from build123d import *

# Parameters (mm, degrees)
BOSS_EXTRUDE1_DEPTH = 13.85


with BuildPart() as part:
    # Sketch1 → Boss-Extrude1 (new, symmetric)
    with BuildSketch(Plane(origin=(0, 0, 0), x_dir=(0, 0, -1), z_dir=(1, 0, 0))):
        with BuildLine():
            ThreePointArc((74.3, 0), (67.119640803, -31.866029224), (46.966384428, -57.572986146))
            Line((46.966384428, -57.572986146), (47.463876439, -58.070478157))
            ThreePointArc((47.463876439, -58.070478157), (67.76721454, -32.13416614), (75, 0))
            ThreePointArc((75, 0), (50.311529494, 55.621488653), (-7.5, 74.624057783))
            Line((-7.5, 74.624057783), (-7.5, 73.920497834))
            ThreePointArc((-7.5, 73.920497834), (49.815860928, 55.125946704), (74.3, 0))
        make_face()
    extrude(amount=BOSS_EXTRUDE1_DEPTH, both=True)


solid = part.part
For this review, take the finished solid that the model builds, in its own axes (mm). Round coordinates to 2 decimals unless told otherwise and drop trailing zeros. Order: outer loops, then holes, each group sorted by start corner. A loop starts at its lowest first (then second) coordinate and runs counter-clockwise, first axis right, second up. Notation, with made-up numbers: (80, 42.5) -> (98, 42.5) arc R19 cw to (98, 59.5) -> close; hole circle Ø5 at (59, 42.5). An arc over 180 degrees is marked (long way). Write item = value, one per line. Start each with the question number.
1) Take a section at C-C on y = 17. State the section outline as (x, z) points, plus the area to 3 significant figures.
2) To check wall thickness, follow line 1 (Y direction, x = 10.5, z = -17.5); line 2 (Y direction, x = 8.5, z = -19); line 3 (Y direction, x = 6.25, z = -53). State the ranges of each line that lie inside material, in increasing order. Write a range as from..to.
3) Insertion check: pin 1 (12 mm diameter, centred on x = -0.5, z = -27, fed in from -Y); pin 2 (10 mm diameter, centred on y = -39.5, z = -58, fed in from +X); pin 3 (2 mm diameter, centred on x = 0, z = -15, fed in from -Y); pin 4 (4 mm diameter, centred on x = 9, y = 14, fed in from -Z). Each pin has a flat end and moves straight along its axis. Give the tip position at first contact, or say it passes through.
4) Take a section at D-D on z = -27. State the section outline as (x, y) points.
5) Take a section at B-B on x = -9.75. State the section outline as (y, z) points.
Verdict:
q1.outline = (-13.85, -73.05) -> (13.85, -73.05) -> (13.85, -72.33) -> (-13.85, -72.33) -> close
q1.area = 19.9 mm2
q2.line_1 = 72.21..72.93
q2.line_2 = 71.83..72.55
q2.line_3 = -53.07..-52.07, 52.07..53.07
q3.pin_1 = 66.57
q3.pin_2 = 13.85
q3.pin_3 = 72.56
q3.pin_4 = -74.03
q4.outline = (-13.85, 69.22) -> (13.85, 69.22) -> (13.85, 69.97) -> (-13.85, 69.97) -> close
q5.outline = (-58.07, -47.46) arc R75 ccw to (74.62, 7.5) -> (73.92, 7.5) arc R74.3 cw to (-57.57, -46.97) -> close
